The listing builds one solid part. Answer for the finished solid, in the listing's coordinates (mm). Face numbers are marked on the shaded views. A direction names the side the tool comes from. Coordinates: 2 decimals unless noted, no trailing zeros. Loops run counter-clockwise (first coordinate to the right, second up) from the corner with the lowest first, then second, coordinate; pieces in that order, holes last. Notation, with made-up numbers: (24.5, 2) - (57.5, 2) arc R22 ccw to (57.5, 21) - close; hole circle Ø2 at (-26.5, 74.25). An arc over 180 degrees is marked (long way). Use one line per item in the form item = value. Start each with the question number.
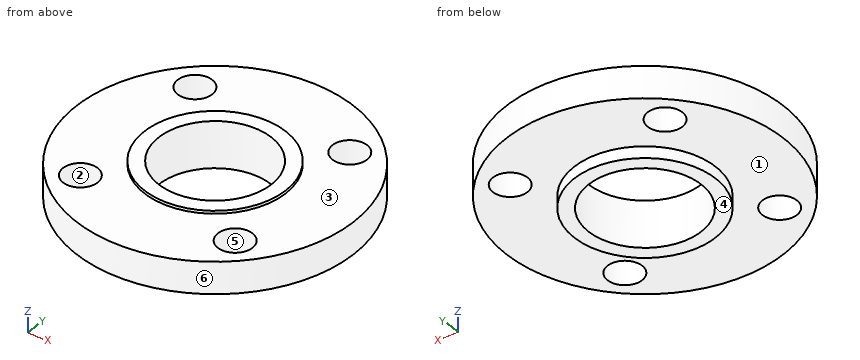
```python
from build123d import *

# Parameters (mm, degrees)
HUB_DIAMETER_R                = 38.862
HUB_DEPTH                     = 25.4
FLANGE_DIAMETER_R             = 76.2
FLANGE_DEPTH                  = 17.4625
REVOLUTION_PROFILE_FOR_BORE_W = 30.988
REVOLUTION_PROFILE_FOR_BORE_H = 228.6
BOLT_DIAMETER_R               = 9.525
BOLT_HOLE_DEPTH               = 111.362652905
BOLT_HOLE_PATTERN_COUNT       = 4
BOLT_HOLE_PATTERN_ANGLE       = 270


with BuildPart() as part:
    # Hub Diameter → Hub (new body)
    with BuildSketch(Plane.XY):
        Circle(HUB_DIAMETER_R)
    extrude(amount=-HUB_DEPTH)

    # Flange Diameter → Flange (add)
    with BuildSketch(Plane.XY.offset(-1.5875)):
        Circle(FLANGE_DIAMETER_R)
    extrude(amount=-FLANGE_DEPTH)

    # Revolution profile for Bore → Bore (revolve, cut)
    with BuildSketch(Plane(origin=(0, 0, 0), x_dir=(1, 0, 0), z_dir=(0, 1, 0))):
        with Locations((15.494, 114.3)):
            Rectangle(REVOLUTION_PROFILE_FOR_BORE_W, REVOLUTION_PROFILE_FOR_BORE_H)
    revolve(axis=Axis((0, 0, 19.52131148), (0, 0, -1)), mode=Mode.SUBTRACT)

    # Bolt Diameter → Bolt Hole (cut, through all)
    with BuildSketch(Plane.XY.offset(-1.5875)):
        with Locations((42.656216575, 42.656216575)):
            Circle(BOLT_DIAMETER_R)
    bolt_hole = extrude(amount=-BOLT_HOLE_DEPTH, mode=Mode.SUBTRACT)

    # Bolt Hole Pattern: Bolt Hole ×4 about axis
    bolt_hole_pattern_axis = Axis((0, 0, -50), (0, 0, 1))
    for i in range(1, BOLT_HOLE_PATTERN_COUNT):
        add(bolt_hole.rotate(bolt_hole_pattern_axis, i * BOLT_HOLE_PATTERN_ANGLE / (BOLT_HOLE_PATTERN_COUNT - 1)), mode=Mode.SUBTRACT)


solid = part.part
```
(1) A cutting plane is placed at A-A (x = 0). Determine the outline of the cut face in (y, z).
(2) For the marked faces 1, 2 and 3, determine the directions among +Z, -Z, +X, -X, +Y, -Y from which every point of the face is accessible in a straight line to the end or side of a thin tool.
(3) A cutting plane is placed at C-C (x = -44.5). Determine the outline of the cut face in (y, z).
(4) A cutting plane is placed at D-D (y = 46.5). Determine the outline of the cut face in (x, z), then the cut area to 3 significant figures.
(5) Determine the mould class of the marked faces 4, 5 and 6 for opening direction Y: +Y half, -Y half, draft (parallel to the pull), parting line (faces both ways), or undercut.
(6) Each of these flat-tipped pins is pushed along its axis until it touches: pin 1 Ø8 at (x, y) = (-26, 35) entering from -Z; pin 2 Ø12 at (x, z) = (52, -16.5) entering from +Y; pin 3 Ø8 at (y, z) = (-12, -8) entering from +X; pin 4 Ø11.5 at (x, y) = (42.66, -42.66) entering from +Z. Where does it stop, or does it pass through?
(7) Find the intervals of material crossed by probe 1 along Y at (x, z) = (0, -15.75); probe 2 along Y at (x, z) = (34.5, -10.5); probe 3 along Y at (x, z) = (47.5, -11.75), in increasing order. Write a range as from..to.
Evaluation:
q1.outline = (-76.2, -19.05) - (-38.86, -19.05) - (-38.86, -25.4) - (-30.99, -25.4) - (-30.99, 0) - (-38.86, 0) - (-38.86, -1.59) - (-76.2, -1.59) - close; (30.99, -25.4) - (38.86, -25.4) - (38.86, -19.05) - (76.2, -19.05) - (76.2, -1.59) - (38.86, -1.59) - (38.86, 0) - (30.99, 0) - close
q2.face_1 = -Z
q2.face_2 = +Z, -Z
q2.face_3 = +Z
q3.outline = (-61.86, -19.05) - (-52, -19.05) - (-52, -1.59) - (-61.86, -1.59) - close; (-33.31, -19.05) - (33.31, -19.05) - (33.31, -1.59) - (-33.31, -1.59) - close; (52, -19.05) - (61.86, -19.05) - (61.86, -1.59) - (52, -1.59) - close
q4.outline = (-60.37, -19.05) - (-51.37, -19.05) - (-51.37, -1.59) - (-60.37, -1.59) - close; (-33.94, -19.05) - (33.94, -19.05) - (33.94, -1.59) - (-33.94, -1.59) - close; (51.37, -19.05) - (60.37, -19.05) - (60.37, -1.59) - (51.37, -1.59) - close
q4.area = 1,500 mm^2
q5.face_4 = draft
q5.face_5 = undercut
q5.face_6 = parting line
q6.pin_1 = -19.05
q6.pin_2 = 60.75
q6.pin_3 = 75.78
q6.pin_4 = through
q7.probe_1 = -76.2..-30.99, 30.99..76.2
q7.probe_2 = -67.94..-47.58, -37.74..37.74, 47.58..67.94
q7.probe_3 = -59.58..-50.86, -34.45..34.45, 50.86..59.58
